```python
from build123d import *

# Parameters (mm, degrees)
SKETCH1_R                 = 8.73125
BOSS_EXTRUDE1_DEPTH       = 4.7625
TAP_DRILL_FOR_8_32_TAP1_D = 3.4544


with BuildPart() as part:
    # Sketch1 → Boss-Extrude1 (new body)
    with BuildSketch(Plane.XY):
        with BuildLine():
            Line((-174.625, 0), (174.625, 0))
            Line((174.625, 0), (160.88501532, -148.391834548))
            ThreePointArc((160.88501532, -148.391834548), (152.705732731, -164.820223727), (135.593202199, -171.45))
            Line((135.593202199, -171.45), (-135.593202199, -171.45))
            ThreePointArc((-135.593202199, -171.45), (-152.705732731, -164.820223727), (-160.88501532, -148.391834548))
            Line((-160.88501532, -148.391834548), (-174.625, 0))
        make_face()
        with Locations(Location((-44.45, -139.7, 0), (0, 0, 180))):
            Circle(SKETCH1_R, mode=Mode.SUBTRACT)
        with Locations(Location((-88.9, -139.7, 0), (0, 0, 180))):
            Circle(SKETCH1_R, mode=Mode.SUBTRACT)
        with Locations(Location((-133.35, -139.7, 0), (0, 0, 180))):
            Circle(SKETCH1_R, mode=Mode.SUBTRACT)
        with Locations(Location((-88.9, -95.25, 0), (0, 0, 180))):
            Circle(SKETCH1_R, mode=Mode.SUBTRACT)
        with Locations(Location((-133.35, -95.25, 0), (0, 0, 180))):
            Circle(SKETCH1_R, mode=Mode.SUBTRACT)
        with Locations(Location((-88.9, -50.8, 0), (0, 0, 180))):
            Circle(SKETCH1_R, mode=Mode.SUBTRACT)
        with Locations(Location((-133.35, -50.8, 0), (0, 0, 180))):
            Circle(SKETCH1_R, mode=Mode.SUBTRACT)
        with Locations(Location((-44.45, -95.25, 0), (0, 0, 180))):
            Circle(SKETCH1_R, mode=Mode.SUBTRACT)
        with Locations(Location((-44.45, -50.8, 0), (0, 0, 180))):
            Circle(SKETCH1_R, mode=Mode.SUBTRACT)
        with Locations(Location((0, -139.7, 0), (0, 0, 180))):
            Circle(SKETCH1_R, mode=Mode.SUBTRACT)
        with Locations(Location((44.45, -139.7, 0), (0, 0, 180))):
            Circle(SKETCH1_R, mode=Mode.SUBTRACT)
        with Locations(Location((88.9, -139.7, 0), (0, 0, 180))):
            Circle(SKETCH1_R, mode=Mode.SUBTRACT)
        with Locations(Location((133.35, -139.7, 0), (0, 0, 180))):
            Circle(SKETCH1_R, mode=Mode.SUBTRACT)
        with Locations(Location((44.45, -95.25, 0), (0, 0, 180))):
            Circle(SKETCH1_R, mode=Mode.SUBTRACT)
        with Locations(Location((88.9, -95.25, 0), (0, 0, 180))):
            Circle(SKETCH1_R, mode=Mode.SUBTRACT)
        with Locations(Location((133.35, -95.25, 0), (0, 0, 180))):
            Circle(SKETCH1_R, mode=Mode.SUBTRACT)
        with Locations(Location((44.45, -50.8, 0), (0, 0, 180))):
            Circle(SKETCH1_R, mode=Mode.SUBTRACT)
        with Locations(Location((88.9, -50.8, 0), (0, 0, 180))):
            Circle(SKETCH1_R, mode=Mode.SUBTRACT)
        with Locations(Location((133.35, -50.8, 0), (0, 0, 180))):
            Circle(SKETCH1_R, mode=Mode.SUBTRACT)
        with Locations(Location((0, -95.25, 0), (0, 0, 180))):
            Circle(SKETCH1_R, mode=Mode.SUBTRACT)
        with Locations(Location((0, -50.8, 0), (0, 0, 180))):
            Circle(SKETCH1_R, mode=Mode.SUBTRACT)
    extrude(amount=BOSS_EXTRUDE1_DEPTH)

    # Tap Drill for #8-32 Tap1 (through all)
    with Locations(Plane.XY.offset(4.7625)):
        with Locations((165.1, -17.78), (-165.1, -17.78)):
            Hole(TAP_DRILL_FOR_8_32_TAP1_D / 2)


solid = part.part
```
Input: part model. Units: mm. Frame: model coordinates. Coordinates: 2 decimals unless noted, no trailing zeros. Loops run counter-clockwise (first coordinate to the right, second up) from the corner with the lowest first, then second, coordinate; pieces in that order, holes last. Notation, with made-up numbers: (7, 51.25) -> (62, 51.25) arc R20 ccw to (62, 72.25) -> close; hole circle Ø4 at (27, -29.75). An arc over 180 degrees is marked (long way). Use a Markdown table: item, result.
1) Cut plane B-B (z = 2.85). Give the number of separate pieces and of enclosed holes in the cut face, then the cut area to 3 significant figures.
Results found:
| item | result |
|---|---|
| separate pieces | 1 |
| enclosed holes | 23 |
| area | 51,900 mm2 |
2) Pull-direction query (Y, two-part tool) for faces 1 (the flat face through (2, -85, 4.762)), 2 (the cylindrical face through (-141.415, -91.906, 2.348)), 3 (the flat face through (167.85, -73.16, 2.35)); classes: released by +Y, released by -Y, zero draft, split by the parting line, or undercut.
Results found:
| item | result |
|---|---|
| face 1 | zero draft |
| face 2 | undercut |
| face 3 | released by -Y |
3) Material intervals for line 1 along Y through (x, z) = (44.45, 1.6); line 2 along Y through (x, z) = (-37, 1.8); line 3 along X through (y, z) = (-121, 0.7), sorted ascending. Write a range as from..to.
Results found:
| item | result |
|---|---|
| line 1 | y = -171.45..-148.43, -130.97..-103.98, -86.52..-59.53, -42.07..0 |
| line 2 | y = -171.45..-144.25, -135.15..-99.8, -90.7..-55.35, -46.25..0 |
| line 3 | x = -163.42..163.42 |
4) Contact query for flat-ended pins moving along their axis: pin 1 (15.5 mm diameter, centred on x = -88.9, y = -139.7, fed in from +Z); pin 2 (22.5 mm diameter, centred on x = 133.35, y = -50.8, fed in from -Z). Output: stop coordinate, or through.
Results found:
| item | result |
|---|---|
| pin 1 | passes through |
| pin 2 | stops at z = 0 |
5) Cut plane A-A (x = 44.45). Return the cut outline in (y, z), then the cut area to 3 significant figures.
Results found:
| item | result |
|---|---|
| outline | (-171.45, 0) -> (-148.43, 0) -> (-148.43, 4.76) -> (-171.45, 4.76) -> close; (-130.97, 0) -> (-103.98, 0) -> (-103.98, 4.76) -> (-130.97, 4.76) -> close; (-86.52, 0) -> (-59.53, 0) -> (-59.53, 4.76) -> (-86.52, 4.76) -> close; (-42.07, 0) -> (0, 0) -> (0, 4.76) -> (-42.07, 4.76) -> close |
| area | 567 mm2 |
6) Cut plane C-C (y = -125.5). Return the cut outline in (x, z).
Results found:
| item | result |
|---|---|
| outline | (-163, 0) -> (163, 0) -> (163, 4.76) -> (-163, 4.76) -> close |
7) Cut plane D-D (y = -82). Return the cut outline in (x, z).
Results found:
| item | result |
|---|---|
| outline | (-167.03, 0) -> (167.03, 0) -> (167.03, 4.76) -> (-167.03, 4.76) -> close |
